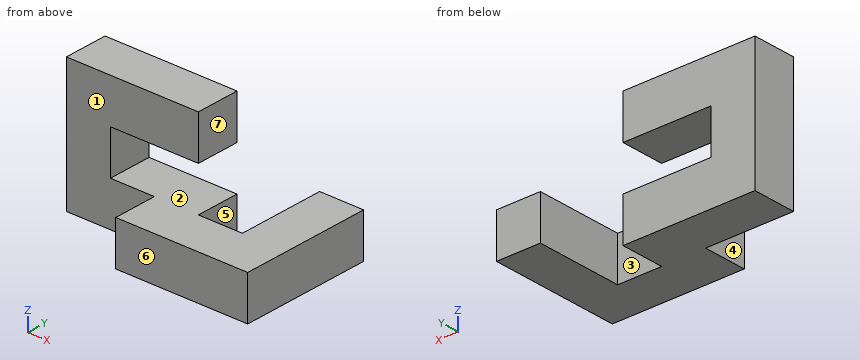
from build123d import *

# Parameters (mm, degrees)
F0_W     = 12.7
F0_H     = 12.7
F1_DEPTH = 12.7
F2_DEPTH = 12.7
F3_DEPTH = 25.4


with BuildPart() as f1:
    # F0 (on Front) → F1 (new body)
    with BuildSketch(Plane.XZ):
        with Locations((-11.356164, 4.188791)):
            Rectangle(F0_W, F0_H)
        with Locations((-24.056164, 4.188791)):
            Rectangle(F0_W, F0_H)
        with Locations((1.343836, 4.188791)):
            Rectangle(F0_W, F0_H)
    extrude(amount=F1_DEPTH)

    # F0 (on Front) → F2 (join)
    with BuildSketch(Plane.XZ):
        with Locations((-24.056164, 4.188791)):
            Rectangle(F0_W, F0_H)
        with Locations((-36.756164, 4.188791)):
            Rectangle(F0_W, F0_H)
        with Locations((-49.456164, 4.188791)):
            Rectangle(F0_W, F0_H)
        with Locations((-49.456164, 16.888791)):
            Rectangle(F0_W, F0_H)
        with Locations((-49.456164, 29.588791)):
            Rectangle(F0_W, F0_H)
        with Locations((-36.756164, 29.588791)):
            Rectangle(F0_W, F0_H)
        with Locations((-24.056164, 29.588791)):
            Rectangle(F0_W, F0_H)
    extrude(amount=-F2_DEPTH)

    # F0 (on Front) → F3 (join)
    with BuildSketch(Plane.XZ):
        with Locations((1.343836, 4.188791)):
            Rectangle(F0_W, F0_H)
    extrude(amount=-F3_DEPTH)


solid = f1.part
Geometry check sheet. Reference: the model listing, model coordinates, mm. Face numbers are marked on the shaded views. A direction names the side the tool comes from. Round coordinates to 2 decimals unless told otherwise and drop trailing zeros. Loops run counter-clockwise (first coordinate to the right, second up) from the corner with the lowest first, then second, coordinate; pieces in that order, holes last.
Item 1: Cross-section at A-A on x = -24. Record the boundary of the cut face in (y, z), then the cut area to 3 significant figures.
Item 2: Thickness scan on line 1 (Z direction, x = -35.5, y = 3); line 2 (X direction, y = -10.5, z = 4); line 3 (Y direction, x = -25.5, z = 33.5). Record the ranges inside material, lowest first.
Item 3: Cross-section at C-C on z = 6. Record the boundary of the cut face in (x, y).
Item 4: Gauge pin test, flat ends, axial feed: pin 1 (19 mm diameter, centred on x = -37, z = 23, fed in from +Y); pin 2 (14 mm diameter, centred on y = 5.5, z = 29.5, fed in from +X); pin 3 (4 mm diameter, centred on y = -8.5, z = 2.5, fed in from -X). Record the tip position at first contact, or that the pin passes through.
Item 5: Cross-section at D-D on x = -37. Record the boundary of the cut face in (y, z), then the cut area to 3 significant figures.
Item 6: Cross-section at B-B on y = 10. Record the boundary of the cut face in (x, z).
Item 7: Access from +Z, -Z, +X, -X, +Y, -Y to the whole of each face (thin tool, end or side, straight path). Record for the marked faces 1, 2 and 3.
Item 8: Mould release check, pull along X, two halves, no side actions. Record for the marked faces 4, 5, 6 and 7: pulls with the +X half, pulls with the -X half, needs draft (parallel to the pull), parting line crosses it, or undercut.
Answer sheet:
1. outline: (-12.7, -2.16) - (12.7, -2.16) - (12.7, 10.54) - (-12.7, 10.54) - close; (0, 23.24) - (12.7, 23.24) - (12.7, 35.94) - (0, 35.94) - close
1. area: 484 mm2
2. line 1: z = -2.16 to 10.54, 23.24 to 35.94
2. line 2: x = -30.41 to 7.69
2. line 3: y = 0 to 12.7
3. outline: (-55.81, 0) - (-30.41, 0) - (-30.41, -12.7) - (7.69, -12.7) - (7.69, 25.4) - (-5.01, 25.4) - (-5.01, 0) - (-17.71, 0) - (-17.71, 12.7) - (-55.81, 12.7) - close
4. pin 1: stops at y = 12.7
4. pin 2: stops at x = -17.71
4. pin 3: stops at x = -30.41
5. outline: (0, -2.16) - (12.7, -2.16) - (12.7, 10.54) - (0, 10.54) - close; (0, 23.24) - (12.7, 23.24) - (12.7, 35.94) - (0, 35.94) - close
5. area: 323 mm2
6. outline: (-55.81, -2.16) - (-17.71, -2.16) - (-17.71, 10.54) - (-43.11, 10.54) - (-43.11, 23.24) - (-17.71, 23.24) - (-17.71, 35.94) - (-55.81, 35.94) - close; (-5.01, -2.16) - (7.69, -2.16) - (7.69, 10.54) - (-5.01, 10.54) - close
7. face 1: +Z, -X, -Y
7. face 2: +X, +Y, -Y
7. face 3: +Z, -Z, +Y
8. face 4: pulls with the -X half
8. face 5: undercut
8. face 6: needs draft
8. face 7: pulls with the +X half
